Geometry check sheet. Reference: the model listing, model coordinates, mm. Face numbers are marked on the shaded views. A direction names the side the tool comes from. Round coordinates to 2 decimals unless told otherwise and drop trailing zeros. Put each result on its own line as item: value. Start each with the question number.
(1) Gauge pin test, flat ends, axial feed: pin 1 (1.2 mm diameter, centred on y = 8.5, z = 4.5, fed in from -X); pin 2 (6 mm diameter, centred on y = 0, z = 0, fed in from +X); pin 3 (2 mm diameter, centred on x = -1.5, z = 4.5, fed in from -Y); pin 4 (1.5 mm diameter, centred on x = -2.5, y = -1, fed in from -Z). Record the tip position at first contact, or that the pin passes through.
(2) Material ranges on probe 1 along Y at (x, z) = (2.2, 0); probe 2 along Y at (x, z) = (-2, -0.25); probe 3 along Z at (x, y) = (-0.5, -6.5), recorded low to high.
(3) Mould release check, pull along Z, two halves, no side actions. Record for the marked faces 1, 2 and 3: pulls with the +Z half, pulls with the -Z half, needs draft (parallel to the pull), parting line crosses it, or undercut.
(4) Tool access check on the marked faces 4 and 5. Record the directions out of +Z, -Z, +X, -X, +Y, -Y that give a thin tool (end or side, any length) a straight path to the whole face; none if there is none.
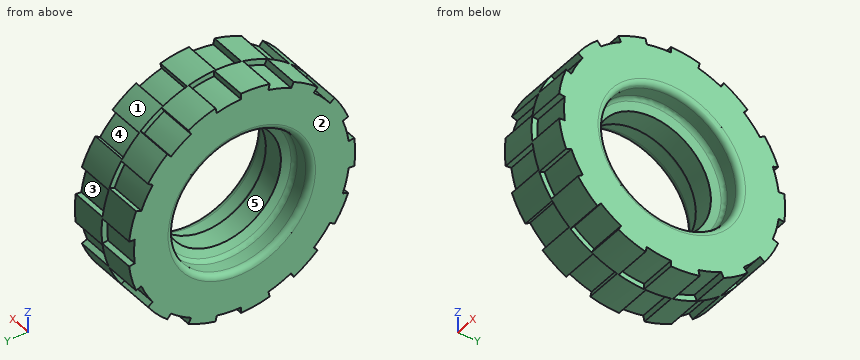
from build123d import *

# Parameters (mm, degrees)
CUT_EXTRUDE1_START = -3.25
CUT_EXTRUDE1_DEPTH = 3.25
CIRPATTERN1_COUNT  = 13
CUT_EXTRUDE2_DEPTH = 3.25
CIRPATTERN2_COUNT  = 13
FILLET1_R          = 0.5


with BuildPart() as part:
    # Sketch1 → Revolve1 (revolve)
    with BuildSketch(Plane.XY, mode=Mode.PRIVATE) as revolve1_sk:
        Polygon((-3.25, 10), (3.25, 10), (3.25, 6), (1.435, 6), (0.915, 5.15), (-0.915, 5.15), (-1.435, 6), (-3.25, 6), align=None)
    revolve(revolve1_sk.sketch.rotate(Axis((0, 0, 0), (1, 0, 0)), 90), axis=Axis((0, 0, 0), (1, 0, 0)))

    # Sketch2 → Cut-Extrude1 (cut)
    with BuildSketch(Plane.ZY.offset(3.25).offset(CUT_EXTRUDE1_START)):
        with BuildLine():
            Line((-1.075430531, 9.438932629), (-1.132032138, 9.935718557))
            ThreePointArc((-1.132032138, 9.935718557), (0, 10), (1.132032138, 9.935718557))
            Line((1.132032138, 9.935718557), (1.075430531, 9.438932629))
            ThreePointArc((1.075430531, 9.438932629), (0, 9.5), (-1.075430531, 9.438932629))
        make_face()
    cut_extrude1 = extrude(amount=CUT_EXTRUDE1_DEPTH, mode=Mode.SUBTRACT)

    # CirPattern1: Cut-Extrude1 ×13 about axis
    cirpattern1_axis = Axis((0, 0, 0), (1, 0, 0))
    for i in range(1, CIRPATTERN1_COUNT):
        add(cut_extrude1.rotate(cirpattern1_axis, i * 360 / CIRPATTERN1_COUNT), mode=Mode.SUBTRACT)

    # Sketch3 → Cut-Extrude2 (cut)
    with BuildSketch(Plane(origin=(3.25, 0, 0), x_dir=(0, 0, -1), z_dir=(1, 0, 0))):
        with BuildLine():
            Line((-3.302885527, 8.907353546), (-3.476721607, 9.376161627))
            ThreePointArc((-3.476721607, 9.376161627), (-2.39296111, 9.709466367), (-1.278436014, 9.917943404))
            Line((-1.278436014, 9.917943404), (-1.214514213, 9.422046233))
            ThreePointArc((-1.214514213, 9.422046233), (-2.273313055, 9.223993048), (-3.302885527, 8.907353546))
        make_face()
    cut_extrude2 = extrude(amount=-CUT_EXTRUDE2_DEPTH, mode=Mode.SUBTRACT)

    # CirPattern2: Cut-Extrude2 ×13 about axis
    cirpattern2_axis = Axis((0, 0, 0), (1, 0, 0))
    for i in range(1, CIRPATTERN2_COUNT):
        add(cut_extrude2.rotate(cirpattern2_axis, i * 360 / CIRPATTERN2_COUNT), mode=Mode.SUBTRACT)

    # Fillet1
    fillet1_edges = [part.edges().sort_by_distance(p)[0] for p in [
        (1.435, 0, -6),
        (3.25, 0, -6),
        (-3.25, 0, -6),
        (-1.435, 0, -6),
    ]]
    fillet(fillet1_edges, radius=FILLET1_R)


solid = part.part
Answers follow:
1. pin 1: stops at x = -3.25
1. pin 2: passes through
1. pin 3: stops at y = -9.37
1. pin 4: stops at z = -10
2. probe 1: y = -9.5 to -6, 6 to 10
2. probe 2: y = -10 to -5.99, 5.99 to 9.5
2. probe 3: z = -7.6 to -7.23, -6.93 to 6.93, 7.23 to 7.6
3. face 1: parting line crosses it
3. face 2: needs draft
3. face 3: undercut
4. face 4: +X
4. face 5: +X, -X
